Work out the finished part from the listing and answer in its coordinate system (mm). A direction names the side the tool comes from. Round coordinates to 2 decimals unless told otherwise and drop trailing zeros. Loops run counter-clockwise (first coordinate to the right, second up) from the corner with the lowest first, then second, coordinate; pieces in that order, holes last.
```python
from build123d import *

# Parameters (mm, degrees)
SKETCH126_W  = 5.7
SKETCH126_H  = 3.8
PAD061_DEPTH = 1.7
SKETCH127_W  = 6.5
SKETCH127_H  = 6.305
PAD062_DEPTH = 1.6
SKETCH128_W  = 6.5
SKETCH128_H  = 7.305
PAD063_DEPTH = 2
CHAMFER_SIZE = 1


with BuildPart() as part:
    # Sketch126 → Pad061 (new body)
    with BuildSketch(Plane.YZ):
        with Locations((-7.89, 12.195)):
            Rectangle(SKETCH126_W, SKETCH126_H)
    extrude(amount=PAD061_DEPTH)

    # Sketch127 → Pad062 (join)
    with BuildSketch(Plane.YZ.offset(1.7)):
        with Locations((-7.89, 10.9425)):
            Rectangle(SKETCH127_W, SKETCH127_H)
    extrude(amount=PAD062_DEPTH)

    # Sketch128 → Pad063 (join)
    with BuildSketch(Plane.YZ):
        with Locations((-7.89, 10.4425)):
            Rectangle(SKETCH128_W, SKETCH128_H)
    extrude(amount=-PAD063_DEPTH)

    # Chamfer
    chamfer_edges = [part.edges().sort_by_distance(p)[0] for p in [
        (-2, -7.89, 14.095),
        (-2, -11.14, 10.4425),
        (-2, -7.89, 6.79),
        (-2, -4.64, 10.4425),
    ]]
    chamfer(chamfer_edges, length=CHAMFER_SIZE)


with BuildPart() as part_1:
    # Body017 placement: moved
    add(part.part.moved(Location((-29.5, 0, 0))))


solid = part_1.part
```
1. Find section C-C (z = 11.75). Write down the section's boundary in (x, y), then the cut area to 3 significant figures.
Answer key:
outline: (-31.5, -10.14) - (-30.5, -11.14) - (-29.5, -11.14) - (-29.5, -10.74) - (-27.8, -10.74) - (-27.8, -11.14) - (-26.2, -11.14) - (-26.2, -4.64) - (-27.8, -4.64) - (-27.8, -5.04) - (-29.5, -5.04) - (-29.5, -4.64) - (-30.5, -4.64) - (-31.5, -5.64) - close
area: 32.1 mm2
2. Given pin 1 (0.5 mm diameter, centred on x = -28.5, z = 13, fed in from +Y); pin 2 (0.8 mm diameter, centred on x = -27, y = -6.5, fed in from -Z); pin 3 (0.8 mm diameter, centred on x = -29, z = 11, fed in from -Y), each flat-ended and moving along its own axis, determine where each tip first touches the part or whether it passes through.
Answer key:
pin 1: stops at y = -5.04
pin 2: stops at z = 7.79
pin 3: stops at y = -10.74
3. Which of the six approach directions +Z, -Z, +X, -X, +Y, -Y give full straight-line access (tool end or side, diameter ignored) to faces 4 (the face through (-27, -8, 7.79)), 5 (the face through (-29, -10.74, 12)), 6 (the face through (-29, -5.04, 12))?
Answer key:
face 4: -Z, +X, +Y, -Y
face 5: +Z, -Z, -Y
face 6: +Z, -Z, +Y
4. Find section B-B (y = -6.25). Write down the section's boundary in (x, z) (3 decimals).
Answer key:
outline: (-31.5, 7.79) - (-30.5, 6.79) - (-29.5, 6.79) - (-29.5, 10.295) - (-27.8, 10.295) - (-27.8, 7.79) - (-26.2, 7.79) - (-26.2, 14.095) - (-30.5, 14.095) - (-31.5, 13.095) - close
5. Find section A-A (z = 8.5). Write down the section's boundary in (x, y).
Answer key:
outline: (-31.5, -10.14) - (-30.5, -11.14) - (-29.5, -11.14) - (-29.5, -4.64) - (-30.5, -4.64) - (-31.5, -5.64) - close; (-27.8, -11.14) - (-26.2, -11.14) - (-26.2, -4.64) - (-27.8, -4.64) - close
6. Determine the mould class of faces 1 (the face through (-31.5, -8, 10)), 2 (the face through (-30, -8, 6.79)), 3 (the face through (-29.5, -8, 9)) for opening direction X: +X half, -X half, draft (parallel to the pull), parting line (faces both ways), or undercut.
Answer key:
face 1: -X half
face 2: draft
face 3: undercut
7. Consider probe 1 along X at (y, z) = (-6.25, 9.25); probe 2 along Y at (x, z) = (-29.45, 12.5); probe 3 along Z at (x, y) = (-29.4, -8) (3 decimals). Determine where each line is inside the solid, lowest interval first.
Answer key:
probe 1: x = -31.5 to -29.5, -27.8 to -26.2
probe 2: y = -10.74 to -5.04
probe 3: z = 10.295 to 14.095
8. Find section D-D (x = -26.6). Write down the section's boundary in (y, z) (3 decimals), then the cut area to 3 significant figures.
Answer key:
outline: (-11.14, 7.79) - (-4.64, 7.79) - (-4.64, 14.095) - (-11.14, 14.095) - close
area: 41.0 mm2
